Check sheet for the modelled part. Datum: model origin and axes. Units: mm. A direction names the side the tool comes from. Give positions to 0.01 mm unless a question says otherwise; leave off trailing zeros. Write each loop counter-clockwise with the first axis right and the second up, starting at its lowest first coordinate (ties: lowest second). Pieces come first, ordered by that corner, then holes. Notation, with made-up numbers: (-13.5, 61) -> (10.5, 61) arc R19 ccw to (10.5, 78) -> close; hole circle Ø10 at (-7.75, 56.5). An arc over 180 degrees is marked (long way). Return JSON: item names as keys, results as strings.
Autodesk Inventor part; units mm, degrees
ref_plane "РабПлоскость1" through (30, 0, 80) normal (1, 0, 0) x (0, 0, -1)
ref_plane "YZ Plane" through (0, 0, 0) normal (1, 0, 0) x (0, 1, 0)
ref_plane "XZ Plane" through (0, 0, 0) normal (0, 1, 0) x (-1, 0, 0)
sketch "Эскиз1" plane through (0, 0, 0) normal (0, 1, 0) x (-1, 0, 0)
  line L0 (-5, 0) -> (-55, 0)
  line L1 (-60, 5) -> (-60, 80)
  line L2 (0, 80) -> (0, 5)
  arc A0 (0, 80) -> (-60, 80) centre (-30, 80) ccw
  circle A1 centre (-30, 80) radius 10
  circle A2 centre (-15, 60) radius 6
  circle A3 centre (-45, 60) radius 6
  line L3 (0, 5) -> (-5, 0)
  line L4 (-60, 5) -> (-55, 0)
  point P0 (0, 0)
  point P1 (-60, 0)
  dimension "d4" = 80
  dimension "d5" = 20
  dimension "d8" = 12
  dimension "d9" = 12
  dimension "d12" = 5
  dimension "d13" = 45
  dimension "d14" = 5
  dimension "d15" = 45
extrude "Выдавливание1" add sketch "Эскиз1" along normal blind 30
sketch "Эскиз2" plane through (0, 30, 0) normal (0, 1, 0) x (1, 0, 0)
  line L0 (0, -20) -> (60, -20)
  line L1 (60, -80) -> (60, -5)
  line L2 (60, -5) -> (55, 0)
  line L3 (60, -5) -> (55, 0)
  line L4 (55, 0) -> (5, 0)
  line L5 (55, 0) -> (5, 0)
  line L6 (5, 0) -> (0, -5)
  line L7 (5, 0) -> (0, -5)
  line L8 (0, -5) -> (0, -20)
  line L9 (0, -5) -> (0, -80)
  point P0 (0, 0)
extrude "Выдавливание2" add sketch "Эскиз2" along normal blind 50
sketch "Эскиз3" plane through (0, 30, 20) normal (0, 0, 1) x (1, 0, 0)
  circle A0 centre (30, 35) radius 10
  line L0 (60, 0) -> (0, 0)
  point P0 (0, -30)
  dimension "d18" = 20
extrude "Выдавливание3" cut sketch "Эскиз3" against normal blind 50
ref_plane "РабПлоскость1" through (30, 0, 80) normal (1, 0, 0) x (0, 0, -1)
sketch "Эскиз6" plane through (30, 0, 80) normal (1, 0, 0) x (0, 0, -1)
  line L0 (60, 30) -> (0, 30)
  line L1 (40, 30) -> (60, 30)
  line L2 (60, 30) -> (60, 50)
  line L3 (60, 30) -> (60, 80)
  line L4 (60, 50) -> (40, 30)
  point P0 (80, 0)
  dimension "d26" = 20
extrude "Выдавливание4" add sketch "Эскиз6" along normal mid plane 12
sketch "Эскиз7" plane through (0, 30, 0) normal (0, 1, 0) x (1, 0, 0)
  line L0 (30, -60) -> (71.6431, -60)
  line L1 (71.6431, -60) -> (71.6431, -124.6271)
  line L2 (71.6431, -124.6271) -> (30, -124.6271)
  line L3 (30, -124.6271) -> (30, -60)
  point P0 (0, 0)
extrude "Выдавливание5" cut sketch "Эскиз7" against normal blind 50
equation "\"d15\" = d13"
(1) Depth check by flat-ended pin: pin 1 Ø10 at (y, z) = (14, 31.5) entering from -X; pin 2 Ø3 at (y, z) = (15.5, 67) entering from +X; pin 3 Ø16 at (y, z) = (42, 33) entering from -X; pin 4 Ø4 at (x, y) = (11, 12.5) entering from +Z. Enter the tip coordinate at first touch or a pass-through.
Reply:
{"pin 1": "x = 0", "pin 2": "x = 30", "pin 3": "x = 24", "pin 4": "z = 104.72"}
(2) Cross-section at C-C on z = 8. Enter the section's corners in (x, y).
Reply:
{"outline": "(0, 0) -> (60, 0) -> (60, 80) -> (0, 80) -> close; hole circle Ø20 at (30, 65)"}
(3) Cross-section at A-A on y = 18.5. Enter the section's corners in (x, z), then the cut area to 3 significant figures.
Reply:
{"outline": "(0, 5) -> (5, 0) -> (55, 0) -> (60, 5) -> (60, 60) -> (51, 60) arc R6 cw to (39, 60) -> (30, 60) -> (30, 70) arc R10 cw to (30, 90) -> (30, 110) arc R30 ccw to (0, 80) -> close; hole circle Ø12 at (15, 60)", "area": "4,560 mm^2"}
(4) Cross-section at D-D on y = 66.5. Enter the section's corners in (x, z), then the cut area to 3 significant figures.
Reply:
{"outline": "(0, 5) -> (5, 0) -> (20.11, 0) -> (20.11, 20) -> (0, 20) -> close; (39.89, 0) -> (55, 0) -> (60, 5) -> (60, 20) -> (39.89, 20) -> close", "area": "780 mm^2"}
(5) Set-up check for faces 1 (the flat face through (29.6, 54.6, 20)), 2 (the flat face through (36, 36, 26)), 3 (the flat face through (55, 15, 60)), 4 (the flat face through (24, 36, 26)): record each of +Z, -Z, +X, -X, +Y, -Y from which the full face is reachable in a straight line by a thin tool's end or side.
Reply:
{"face 1": "+Z, +Y", "face 2": "+Z, +X, +Y", "face 3": "+Z, +X, +Y, -Y", "face 4": "+Z, -X, +Y"}
(6) Thickness scan on L1, parallel to Y at x = 30, z = 16; L2, parallel to Y at x = 51, z = 25; L3, parallel to Z at x = 11.5, y = 36. Record the ranges inside material, lowest first.
Reply:
{"L1": "0 to 55, 75 to 80", "L2": "0 to 30", "L3": "0 to 20"}
(7) Cross-section at B-B on x = 31.5. Enter the section's corners in (y, z), then the cut area to 3 significant figures.
Reply:
{"outline": "(0, 0) -> (55.11, 0) -> (55.11, 20) -> (50, 20) -> (30, 40) -> (30, 60) -> (0, 60) -> close; (74.89, 0) -> (80, 0) -> (80, 20) -> (74.89, 20) -> close", "area": "2,600 mm^2"}
(8) Release check for a two-part mould opening along X. For faces 5 (the flat face through (30, 40, 30)), 6 (the cylindrical face through (45, 15, 54)), 7 (the cylindrical face through (20, 15, 80)) record: pulls with the +X half, pulls with the -X half, needs draft (parallel to the pull), parting line crosses it, or undercut.
Reply:
{"face 5": "needs draft", "face 6": "undercut", "face 7": "pulls with the +X half"}
